```python
from build123d import *

# Parameters (mm, degrees)
F0_R     = 175
F1_DEPTH = 35
F3_D     = 50
F4_SIZE  = 5
F6_DEPTH = 10.21899


with BuildPart() as f1:
    # F0 (on Front) → F1 (new body)
    with BuildSketch(Plane.XZ):
        Circle(F0_R)
    extrude(amount=F1_DEPTH)

    # F3 (through all)
    with Locations(Plane.XZ.offset(35)):
        with Locations((0, 0)):
            Hole(F3_D / 2)

    # F4
    f4_edges = [f1.edges().sort_by_distance(p)[0] for p in [
        (-175, -35, 0),
        (-175, 0, 0),
    ]]
    chamfer(f4_edges, length=F4_SIZE)

    # F5 (on face) → F6 (cut)
    with BuildSketch(Plane.XZ.offset(35)):
        with BuildLine():
            Line((-155.457131, 0), (-130.677676, 0))
            ThreePointArc((-130.677676, 0), (0, 130.677676), (130.677676, 0))
            Line((130.677676, 0), (155.457131, 0))
            ThreePointArc((155.457131, 0), (0, 155.457131), (-155.457131, 0))
        make_face()
    extrude(amount=-F6_DEPTH, mode=Mode.SUBTRACT)


solid = f1.part
```
Geometry: final body of the model. Coordinates: model frame, mm. A direction names the side the tool comes from. Round coordinates to 2 decimals unless told otherwise and drop trailing zeros. Write each loop counter-clockwise with the first axis right and the second up, starting at its lowest first coordinate (ties: lowest second). Pieces come first, ordered by that corner, then holes. Notation, with made-up numbers: (-24, 14) -> (-14, 14) arc R10 ccw to (-14, 23) -> close; hole circle Ø8 at (47.5, 86.25). An arc over 180 degrees is marked (long way). Return JSON: item names as keys, results as strings.
Q1. First-contact query: pin 1 Ø4 at (x, y) = (-41, -13.5) entering from +Z; pin 2 Ø5 at (x, y) = (85.5, -23) entering from -Z; pin 3 Ø3 at (x, y) = (141.5, -29.5) entering from +Z; pin 4 Ø12 at (x, z) = (-10.5, -9) entering from -Y. Flat tips, straight axial feed; report the tip coordinate or a pass-through.
From the geometry:
{"pin 1": "z = 170.6", "pin 2": "z = -154.06", "pin 3": "z = 105", "pin 4": "through"}
Q2. Section B-B on y = -19.5. Return the cut outline in (x, z).
From the geometry:
{"outline": "circle Ø350 at (0, 0); hole circle Ø50 at (0, 0)"}
Q3. Set-up query: faces 4 (the flat face through (-2, -35, -35)), 5 (the cylindrical face through (-2.874, -29.962, 130.646)). Return all of +Z, -Z, +X, -X, +Y, -Y with unobstructed straight access to the full face (end or side cutting, diameter ignored); none if empty.
From the geometry:
{"face 4": "+Z, -Z, +X, -X, -Y", "face 5": "-Y"}
Q4. Mould query, pull axis X, two halves, no side actions, for faces 1 (the cylindrical face through (-23.846, -17.255, 7.509)), 2 (the flat face through (-2, 0, -35)), 3 (the conical face through (-135.099, -0.243, -103.59)). Classes: +X half, -X half, draft (parallel to the pull), parting line (faces both ways), or undercut.
From the geometry:
{"face 1": "undercut", "face 2": "draft", "face 3": "parting line"}
Q5. Section A-A on x = 0. Return the cut outline in (y, z), and give its area (3 significant figures).
From the geometry:
{"outline": "(-35, -170) -> (-30, -175) -> (-5, -175) -> (0, -170) -> (0, -25) -> (-35, -25) -> close; (-35, 25) -> (0, 25) -> (0, 170) -> (-5, 175) -> (-30, 175) -> (-35, 170) -> (-35, 155.46) -> (-24.78, 155.46) -> (-24.78, 130.68) -> (-35, 130.68) -> close", "area": "10,200 mm2"}
Q6. Ray query, line 1 (Z direction, x = 0, y = -27); line 2 (Z direction, x = 0, y = -8); line 3 (Y direction, x = -24, z = 132). Return the intervals inside material, ascending.
From the geometry:
{"line 1": "-175 to -25, 25 to 130.68, 155.46 to 175", "line 2": "-175 to -25, 25 to 175", "line 3": "-24.78 to 0"}
